```python
from build123d import *

# Parameters (mm, degrees)
CUT_EXTRUDE1_DEPTH = 2
FILLET1_R          = 0.5
FILLET2_R          = 0.5


with BuildPart() as part:
    # Sketch1 → Revolve1 (revolve)
    with BuildSketch(Plane.XY):
        Polygon((0, 0), (7, 0), (7, 6), (4, 6), (4, 15), (3, 15), (3, 22), (0, 22), align=None)
    revolve(axis=Axis((0, 22, 0), (0, -1, 0)))

    # Sketch2 → Cut-Extrude1 (cut)
    with BuildSketch(Plane.XZ):
        Polygon((0, -4.618802154), (4, -2.309401077), (4, 2.309401077), (0, 4.618802154), (-4, 2.309401077), (-4, -2.309401077), align=None)
    extrude(amount=-CUT_EXTRUDE1_DEPTH, mode=Mode.SUBTRACT)

    # Fillet1
    fillet1_edges = [part.edges().sort_by_distance(p)[0] for p in [
        (-4, 6, 0),
    ]]
    fillet(fillet1_edges, radius=FILLET1_R)

    # Fillet2
    fillet2_edges = [part.edges().sort_by_distance(p)[0] for p in [
        (-3, 15, 0),
    ]]
    fillet(fillet2_edges, radius=FILLET2_R)


solid = part.part
```
Geometry: final body of the model. Coordinates: model frame, mm. A direction names the side the tool comes from. Round coordinates to 2 decimals unless told otherwise and drop trailing zeros. Write each loop counter-clockwise with the first axis right and the second up, starting at its lowest first coordinate (ties: lowest second). Pieces come first, ordered by that corner, then holes. Notation, with made-up numbers: (-32, 62) -> (23, 62) arc R23 cw to (23, 98) -> close; hole circle Ø6 at (-26, 72.25). An arc over 180 degrees is marked (long way). Return JSON: item names as keys, results as strings.
Q1. Section A-A on z = 0. Return the cut outline in (x, y), and give its area (3 significant figures).
From the geometry:
{"outline": "(-7, 0) -> (-4, 0) -> (-4, 2) -> (4, 2) -> (4, 0) -> (7, 0) -> (7, 6) -> (4.5, 6) arc R0.5 cw to (4, 6.5) -> (4, 15) -> (3.5, 15) arc R0.5 cw to (3, 15.5) -> (3, 22) -> (-3, 22) -> (-3, 15.5) arc R0.5 cw to (-3.5, 15) -> (-4, 15) -> (-4, 6.5) arc R0.5 cw to (-4.5, 6) -> (-7, 6) -> close", "area": "182 mm2"}
Q2. Section D-D on y = 16.75. Return the cut outline in (x, z).
From the geometry:
{"outline": "circle Ø6 at (0, 0)"}
Q3. Set-up query: faces 1 (the flat face through (0, 0, -5)), 2 (the cylindrical face through (-0.867, 10.81, -3.905)), 3 (the flat face through (1.97, 0.99, -3.48)). Return all of +Z, -Z, +X, -X, +Y, -Y with unobstructed straight access to the full face (end or side cutting, diameter ignored); none if empty.
From the geometry:
{"face 1": "+Z, -Z, +X, -X, -Y", "face 2": "+Y", "face 3": "-Y"}
Q4. Mould query, pull axis X, two halves, no side actions, for faces 4 (the cylindrical face through (6.466, 3.042, -2.681)), 5 (the flat face through (0, 22, 0)), 6 (the flat face through (2.028, 0.986, 3.448)). Classes: +X half, -X half, draft (parallel to the pull), parting line (faces both ways), or undercut.
From the geometry:
{"face 4": "parting line", "face 5": "draft", "face 6": "undercut"}
Q5. Section C-C on x = 5.5. Return the cut outline in (y, z).
From the geometry:
{"outline": "(0, -4.33) -> (6, -4.33) -> (6, 4.33) -> (0, 4.33) -> close"}
Q6. Ray query, line 1 (Y direction, x = -4.5, z = -3); line 2 (Y direction, x = -2.25, z = 1.75); line 3 (X direction, y = 11.75, z = -0.25). Return the intervals inside material, ascending.
From the geometry:
{"line 1": "0 to 6", "line 2": "2 to 22", "line 3": "-3.99 to 3.99"}
Q7. First-contact query: pin 1 Ø1 at (x, z) = (0.5, -5.5) entering from +Y; pin 2 Ø8 at (y, z) = (2.5, -5.5) entering from +X; pin 3 Ø8 at (x, y) = (2, 17.5) entering from +Z. Flat tips, straight axial feed; report the tip coordinate or a pass-through.
From the geometry:
{"pin 1": "y = 6", "pin 2": "x = 6.84", "pin 3": "z = 4"}
Q8. Section B-B on y = 9.25. Return the cut outline in (x, z).
From the geometry:
{"outline": "circle Ø8 at (0, 0)"}
